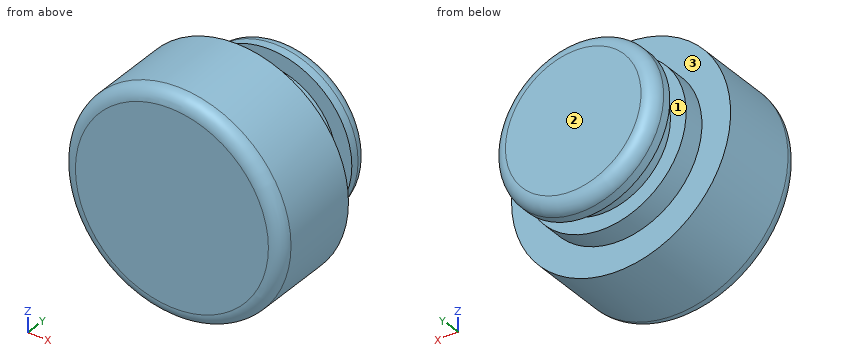
from build123d import *

# Parameters (mm, degrees)
FILLET1_R = 1
FILLET2_R = 1


with BuildPart() as part:
    # Sketch1 → Revolve1 (revolve)
    with BuildSketch(Plane.XY):
        Polygon((0, 0), (0, 12), (6.2, 12), (6.2, 10.35), (5, 10.35), (5, 8.65), (6.2, 8.65), (6.2, 7), (8.4, 7), (8.4, 0), align=None)
    revolve(axis=Axis((0, 0, 0), (0, 1, 0)))

    # Fillet1
    fillet1_edges = [part.edges().sort_by_distance(p)[0] for p in [
        (-6.2, 12, 0),
    ]]
    fillet(fillet1_edges, radius=FILLET1_R)

    # Fillet2
    fillet2_edges = [part.edges().sort_by_distance(p)[0] for p in [
        (-8.4, 0, 0),
    ]]
    fillet(fillet2_edges, radius=FILLET2_R)


solid = part.part
Check sheet for the modelled part. Datum: model origin and axes. Units: mm. Face numbers are marked on the shaded views. A direction names the side the tool comes from. Give positions to 0.01 mm unless a question says otherwise; leave off trailing zeros. Order: outer loops, then holes, each group sorted by start corner. A loop starts at its lowest first (then second) coordinate and runs counter-clockwise, first axis right, second up. Notation, with made-up numbers: (9.25, 39.25) - (50.25, 39.25) arc R7 ccw to (50.25, 48.25) - close; hole circle Ø1 at (-16, -24). An arc over 180 degrees is marked (long way). Answer as CSV lines item,"result".
1. Go/stop test with a flat-tipped pin: P1, Ø2, axis at y = 4.5, z = 2.5, coming from the -X side (3 decimals). Record where the tip stops, or that it passes through.
Result sheet:
P1,"x = -8.265"
2. Scan lines: probe 1 along Y at (x, z) = (-3, 6.5); probe 2 along Y at (x, z) = (-5.75, -1); probe 3 along Z at (x, y) = (3.25, 10.5). Record each from-to range of solid material in increasing order. Write a range as from..to.
Result sheet:
probe 1,"0..7"
probe 2,"0..8.65, 10.35..11.77"
probe 3,"-5.28..5.28"
3. Section check B-B (z = 0). Record the boundary of the cut face in (x, y), then the cut area to 3 significant figures.
Result sheet:
outline,"(-8.4, 1) arc R1 ccw to (-7.4, 0) - (7.4, 0) arc R1 ccw to (8.4, 1) - (8.4, 7) - (6.2, 7) - (6.2, 8.65) - (5, 8.65) - (5, 10.35) - (6.2, 10.35) - (6.2, 11) arc R1 ccw to (5.2, 12) - (-5.2, 12) arc R1 ccw to (-6.2, 11) - (-6.2, 10.35) - (-5, 10.35) - (-5, 8.65) - (-6.2, 8.65) - (-6.2, 7) - (-8.4, 7) - close"
area,"175 mm²"
4. Section check A-A (x = 0). Record the boundary of the cut face in (y, z).
Result sheet:
outline,"(0, -7.4) arc R1 ccw to (1, -8.4) - (7, -8.4) - (7, -6.2) - (8.65, -6.2) - (8.65, -5) - (10.35, -5) - (10.35, -6.2) - (11, -6.2) arc R1 ccw to (12, -5.2) - (12, 5.2) arc R1 ccw to (11, 6.2) - (10.35, 6.2) - (10.35, 5) - (8.65, 5) - (8.65, 6.2) - (7, 6.2) - (7, 8.4) - (1, 8.4) arc R1 ccw to (0, 7.4) - close"
5. Tool access check on the marked faces 1, 2 and 3. Record the directions out of +Z, -Z, +X, -X, +Y, -Y that give a thin tool (end or side, any length) a straight path to the whole face; none if there is none.
Result sheet:
face 1,"none"
face 2,"+Z, -Z, +X, -X, +Y"
face 3,"+Y"
6. Section check D-D (y = 6.5). Record the boundary of the cut face in (x, z).
Result sheet:
outline,"circle Ø16.8 at (0, 0)"
7. Section check C-C (y = 9.5). Record the boundary of the cut face in (x, z), then the cut area to 3 significant figures.
Result sheet:
outline,"circle Ø10 at (0, 0)"
area,"78.5 mm²"
